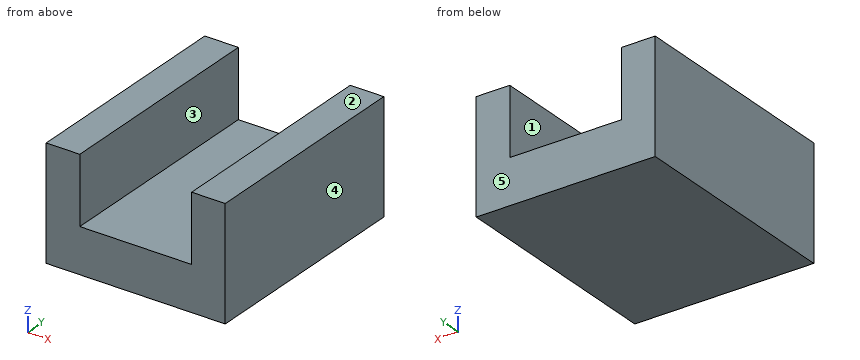
Solid Edge part; units mm, degrees
sketch "Sketch1" plane through (0, 0, 0) normal (0, -1, 0) x (1, 0, 0)
  line L0 (-40, -25) -> (40, -25)
  line L1 (40, -25) -> (40, 25)
  line L2 (40, 25) -> (-40, 25)
  line L3 (-40, 25) -> (-40, -25)
  dimension "D1" = 40
  dimension "D2" = 40
extrude "Protrusion1" add sketch "Sketch1" along normal mid plane 100
sketch "Sketch2" plane through (0, -50, 0) normal (0, -1, 0) x (1, 0, 0)
  line L0 (-25, 25) -> (25, 25)
  line L1 (25, 25) -> (25, -5)
  line L2 (25, -5) -> (-25, -5)
  line L3 (-25, -5) -> (-25, 25)
  dimension "D1" = 25
extrude "Cutout1" cut sketch "Sketch2" against normal through all
properties material "알루미늄, 1060"
Geometry check sheet. Reference: the model listing, model coordinates, mm. Face numbers are marked on the shaded views. A direction names the side the tool comes from. Coordinates: 2 decimals unless noted, no trailing zeros. Order: outer loops, then holes, each group sorted by start corner. A loop starts at its lowest first (then second) coordinate and runs counter-clockwise, first axis right, second up. Notation, with made-up numbers: (81, 38.5) - (125, 38.5) arc R34 ccw to (125, 76.5) - close; hole circle Ø4 at (29, -4.75). An arc over 180 degrees is marked (long way). Use one line per item in the form item = value.
1. Gauge pin test, flat end, axial feed: pin 1 (25 mm diameter, centred on x = -11.5, y = -8, fed in from +Z). Record the tip position at first contact, or that the pin passes through.
Here are the results:
pin_1 = -5
2. Draft check along X on the marked faces 3, 4 and 5. Enter one of: pulls with the +X half, pulls with the -X half, needs draft (parallel to the pull), parting line crosses it, or undercut.
Here are the results:
face_3 = undercut
face_4 = pulls with the +X half
face_5 = needs draft
3. Section check A-A (z = 9.5). Record the boundary of the cut face in (x, y).
Here are the results:
outline = (-40, -50) - (-25, -50) - (-25, 50) - (-40, 50) - close; (25, -50) - (40, -50) - (40, 50) - (25, 50) - close
4. Access from +Z, -Z, +X, -X, +Y, -Y to the whole of each face (thin tool, end or side, straight path). Record for the marked faces 1 and 2.
Here are the results:
face_1 = +Z, +Y, -Y
face_2 = +Z, +X, -X, +Y, -Y
5. Section check C-C (x = -1.5). Record the boundary of the cut face in (y, z).
Here are the results:
outline = (-50, -25) - (50, -25) - (50, -5) - (-50, -5) - close
6. Section check B-B (y = -43). Record the boundary of the cut face in (x, z), then the cut area to 3 significant figures.
Here are the results:
outline = (-40, -25) - (40, -25) - (40, 25) - (25, 25) - (25, -5) - (-25, -5) - (-25, 25) - (-40, 25) - close
area = 2,500 mm²
7. Scan lines: line 1 (X direction, y = -0.5, z = 23); line 2 (Z direction, x = 19, y = 39). Record each from-to range of solid material in increasing order.
Here are the results:
line_1 = -40 to -25, 25 to 40
line_2 = -25 to -5
